Verification items for the finished model (mm, model axes). A direction names the side the tool comes from. Coordinates: 2 decimals unless noted, no trailing zeros. Order: outer loops, then holes, each group sorted by start corner. A loop starts at its lowest first (then second) coordinate and runs counter-clockwise, first axis right, second up. Notation, with made-up numbers: M 23,40 L 78,40 A14 ccw 78,61 Z; hole C 73,22 d3. An arc over 180 degrees is marked long. Answer as a JSON object with one key per item and string values. Group by question number.
(1) Cross-section at A-A (y = 0.5). Enter the section's corners in (x, z), plus the area to 3 significant figures.
(2) Gauge pin test, flat ends, axial feed: pin 1 Ø1 at (x, z) = (-12.5, 0.5) entering from -Y; pin 2 Ø1.4 at (x, z) = (-14.5, 1) entering from -Y; pin 3 Ø7.5 at (x, y) = (0, -18.5) entering from -Z; pin 4 Ø1.5 at (x, y) = (-2, 2.5) entering from +Z. Record the tip position at first contact, or that the pin passes through.
(3) Material ranges on line 1 (Y direction, x = 0, z = 0.65); line 2 (Y direction, x = -5.5, z = 0.65); line 3 (X direction, y = -1, z = 0.55), recorded low to high.
(4) Cross-section at B-B (x = -1.75). Enter the section's corners in (y, z).
(5) Access from +Z, -Z, +X, -X, +Y, -Y to the whole of each face (thin tool, end or side, straight path). Record for faces 1 (the face through (-14, 10, 1)), 2 (the face through (-16, 0, 1)), 3 (the face through (0, -22.5, 1)), 4 (the face through (-7, -5.5, 1)).
(6) Mould release check, pull along X, two halves, no side actions. Record for faces 5 (the face through (-7.84, 14.01, 1.52)), 6 (the face through (-2, 0, 0)), 7 (the face through (0.52, -20.843, 1.479)): released by +X, released by -X, zero draft, split by the parting line, or undercut.
(7) Cross-section at D-D (z = 1.6). Count the separate pieces of the cut face and the enclosed holes in it, plus the area to 3 significant figures.
(8) Cross-section at C-C (x = -14.5). Enter the section's corners in (y, z).
from build123d import *

# Parameters (mm, degrees)
EXTRUDE_1_DEPTH    = 3
HOLE_WIZARD_M4_1_D = 4.8
SKETCH_5_W         = 5
SKETCH_5_H         = 11
EXTRUDE_2_DEPTH    = 0.8
FILLET_6_R         = 2


with BuildPart() as part:
    # ｽｹｯﾁ1 → ﾎﾞｽ - 押し出し1 (new body)
    with BuildSketch(Plane(origin=(0, 0, 0), x_dir=(0, 1, 0), z_dir=(0, 0, 1))):
        with BuildLine():
            Line((-22.5, 7.5), (-22.5, -7.5))
            Line((-22.5, -7.5), (22.5, -7.5))
            Line((22.5, -7.5), (22.5, 7.5))
            Line((22.5, 7.5), (13.5, 7.5))
            ThreePointArc((13.5, 7.5), (10, 4), (6.5, 7.5))
            Line((6.5, 7.5), (5.5, 7.5))
            Line((5.5, 7.5), (5.5, -1))
            Line((5.5, -1), (-5.5, -1))
            Line((-5.5, -1), (-5.5, 7.5))
            Line((-5.5, 7.5), (-6.5, 7.5))
            ThreePointArc((-6.5, 7.5), (-10, 4), (-13.5, 7.5))
            Line((-13.5, 7.5), (-22.5, 7.5))
        make_face()
        with BuildLine():
            Line((-10, 17.5), (-10, 11))
            ThreePointArc((-10, 11), (-7.525126266, 9.974873734), (-6.5, 7.5))
            Line((-6.5, 7.5), (-5.5, 7.5))
            Line((-5.5, 7.5), (-5.5, 16))
            Line((-5.5, 16), (5.5, 16))
            Line((5.5, 16), (5.5, 7.5))
            Line((5.5, 7.5), (6.5, 7.5))
            ThreePointArc((6.5, 7.5), (7.525126266, 9.974873734), (10, 11))
            Line((10, 11), (10, 17.5))
            Line((10, 17.5), (-10, 17.5))
        make_face()
        with BuildLine():
            ThreePointArc((-6.5, 7.5), (-7.525126266, 9.974873734), (-10, 11))
            Line((-10, 11), (-10, 9.05))
            ThreePointArc((-10, 9.05), (-8.903984489, 8.596015511), (-8.45, 7.5))
            Line((-8.45, 7.5), (-6.5, 7.5))
        make_face()
        with BuildLine():
            ThreePointArc((-10, 11), (-12.474873734, 9.974873734), (-13.5, 7.5))
            Line((-13.5, 7.5), (-11.55, 7.5))
            ThreePointArc((-11.55, 7.5), (-11.096015511, 8.596015511), (-10, 9.05))
            Line((-10, 9.05), (-10, 11))
        make_face()
        with BuildLine():
            Line((-11.55, 7.5), (-13.5, 7.5))
            ThreePointArc((-13.5, 7.5), (-10, 4), (-6.5, 7.5))
            Line((-6.5, 7.5), (-8.45, 7.5))
            ThreePointArc((-8.45, 7.5), (-10, 5.95), (-11.55, 7.5))
        make_face()
        with BuildLine():
            Line((10, 9.05), (10, 11))
            ThreePointArc((10, 11), (7.525126266, 9.974873734), (6.5, 7.5))
            Line((6.5, 7.5), (8.45, 7.5))
            ThreePointArc((8.45, 7.5), (8.903984489, 8.596015511), (10, 9.05))
        make_face()
        with BuildLine():
            Line((11.55, 7.5), (13.5, 7.5))
            ThreePointArc((13.5, 7.5), (12.474873734, 9.974873734), (10, 11))
            Line((10, 11), (10, 9.05))
            ThreePointArc((10, 9.05), (11.096015511, 8.596015511), (11.55, 7.5))
        make_face()
        with BuildLine():
            ThreePointArc((6.5, 7.5), (10, 4), (13.5, 7.5))
            Line((13.5, 7.5), (11.55, 7.5))
            ThreePointArc((11.55, 7.5), (10, 5.95), (8.45, 7.5))
            Line((8.45, 7.5), (6.5, 7.5))
        make_face()
    extrude(amount=EXTRUDE_1_DEPTH)

    # M4 すきま穴1 (through all)
    with Locations(Plane.XY.offset(3)):
        with Locations((0, -18.5), (0, 18.5)):
            Hole(HOLE_WIZARD_M4_1_D / 2)

    # ｽｹｯﾁ5 → ﾎﾞｽ - 押し出し2 (add)
    with BuildSketch(Plane(origin=(0, 0, 0), x_dir=(1, 0, 0), z_dir=(0, 0, -1))):
        with Locations((-1.5, 0)):
            Rectangle(SKETCH_5_W, SKETCH_5_H)
    extrude(amount=-EXTRUDE_2_DEPTH)

    # ﾌｨﾚｯﾄ6
    fillet_6_edges = [part.edges().sort_by_distance(p)[0] for p in [
        (-16, -5.5, 1.5),
        (1, -5.5, 1.9),
        (1, 5.5, 1.9),
        (-16, 5.5, 1.5),
        (-7.5, 13.5, 1.5),
        (-7.5, 22.5, 1.5),
        (7.5, 22.5, 1.5),
        (7.5, -22.5, 1.5),
        (-7.5, -22.5, 1.5),
        (-7.5, -13.5, 1.5),
        (-11, -10, 1.5),
        (-17.5, -10, 1.5),
        (-17.5, 10, 1.5),
        (-11, 10, 1.5),
    ]]
    fillet(fillet_6_edges, radius=FILLET_6_R)


solid = part.part
Taken from the geometry:
{
 "1": {"outline": "M -17.5,0 L -16,0 L -16,3 L -17.5,3 Z; M -4,0 L 7.5,0 L 7.5,3 L 1,3 L 1,0.8 L -4,0.8 Z", "area": "28.0 mm²"},
 "2": {"pin 1": "stops at y = -10.1", "pin 2": "stops at y = -10", "pin 3": "stops at z = 0", "pin 4": "stops at z = 0.8"},
 "3": {"line 1": "y = -22.5 to -20.9, -16.1 to 16.1, 20.9 to 22.5", "line 2": "y = -22.5 to -5.5, 5.5 to 22.5", "line 3": "x = -17.5 to -16, -4 to 7.5"},
 "4": {"outline": "M -22.5,0 L -20.14,0 L -20.14,3 L -22.5,3 Z; M -16.86,0 L 16.86,0 L 16.86,3 L 5.5,3 L 5.5,0.8 L -5.5,0.8 L -5.5,3 L -16.86,3 Z; M 20.14,0 L 22.5,0 L 22.5,3 L 20.14,3 Z"},
 "5": {"face 1": "+Z, -Z, -X, +Y", "face 2": "+Z, -Z", "face 3": "+Z, -Z, +X, -X, -Y", "face 4": "+Z"},
 "6": {"face 5": "released by -X", "face 6": "zero draft", "face 7": "undercut"},
 "7": {"separate pieces": "1", "enclosed holes": "5", "area": "656 mm²"},
 "8": {"outline": "M -10,0 L -5.44,0 L -5.44,3 L -10,3 Z; M 5.44,0 L 10,0 L 10,3 L 5.44,3 Z"}
}
